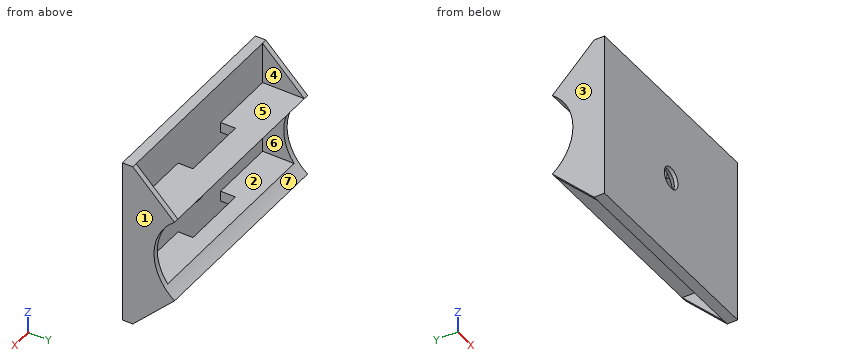
```python
from build123d import *

# Parameters (mm, degrees)
SKETCH4_W           = 25.4
SKETCH4_H           = 1.5875
SKETCH4_W_2         = 1.5875
SKETCH4_H_2         = 6.35
BOSS_EXTRUDE2_DEPTH = 31.75
SKETCH5_W           = 9.525
SKETCH5_H           = 6.35
BOSS_EXTRUDE3_DEPTH = 0.79375
BOSS_EXTRUDE4_DEPTH = 0.79375
SKETCH7_W           = 10.16
SKETCH7_H           = 2.260476196
CUT_EXTRUDE1_DEPTH  = 38.867781903
CUT_EXTRUDE2_REACH  = 43.427
SKETCH8_R           = 8.011204241


with BuildPart() as part:
    # Sketch4 → Boss-Extrude2 (new body)
    with BuildSketch(Plane(origin=(0, 0, 0), x_dir=(0, 0, -1), z_dir=(1, 0, 0))):
        with Locations((12.7, 0.79375)):
            Rectangle(SKETCH4_W, SKETCH4_H)
        with Locations((7.14375, 4.7625)):
            Rectangle(SKETCH4_W_2, SKETCH4_H_2)
        with Locations((18.25625, 4.7625)):
            Rectangle(SKETCH4_W_2, SKETCH4_H_2)
    extrude(amount=BOSS_EXTRUDE2_DEPTH)

    # Sketch5 → Boss-Extrude3 (add)
    with BuildSketch(Plane(origin=(31.75, 0, 0), x_dir=(0, 0, -1), z_dir=(1, 0, 0))):
        Polygon((6.35, 7.9375), (0, 1.5875), (6.35, 1.5875), align=None)
        with Locations((12.7, 4.7625)):
            Rectangle(SKETCH5_W, SKETCH5_H)
        Polygon((19.05, 7.9375), (19.05, 1.5875), (25.4, 1.5875), align=None)
    extrude(amount=-BOSS_EXTRUDE3_DEPTH)

    # Sketch6 → Boss-Extrude4 (add)
    with BuildSketch(Plane.ZY):
        Polygon((-25.4, 1.5875), (0, 1.5875), (-6.35, 7.9375), (-19.05, 7.9375), align=None)
    extrude(amount=-BOSS_EXTRUDE4_DEPTH)

    # Sketch7 → Cut-Extrude1 (cut, through all)
    with BuildSketch(Plane.XY.offset(-6.35)):
        with Locations((15.875, 2.717738098)):
            Rectangle(SKETCH7_W, SKETCH7_H)
    extrude(amount=-CUT_EXTRUDE1_DEPTH, mode=Mode.SUBTRACT)

    # Sketch8 → Cut-Extrude2 (cut, up to next)
    with BuildSketch(Plane(origin=(31.75, 0, 0), x_dir=(0, 0, -1), z_dir=(1, 0, 0)), mode=Mode.PRIVATE) as cut_extrude2_sk1:
        with Locations((12.7, 12.82185189)):
            Circle(SKETCH8_R)
    cut_extrude2_tool1 = extrude(cut_extrude2_sk1.sketch, amount=-CUT_EXTRUDE2_REACH, mode=Mode.PRIVATE) & part.part
    add(cut_extrude2_tool1.solids().sort_by_distance((31.75, 12.821852, -12.7))[0], mode=Mode.SUBTRACT)

    # Sketch10 → CSK for #4 Flat Head Machine Screw (100)1 (revolve, cut)
    with BuildSketch(Plane(origin=(15.887282669, 1.5875, -12.697770178), x_dir=(0, 0, 1), z_dir=(1, 0, 0))):
        Polygon((0, 0), (0, 1.5875), (1.63195, 1.5875), (1.63195, 1.028358553), (2.8575, 0), align=None)
    revolve(axis=Axis((15.887282669, 7.9375, -12.697770178), (0, -1, 0)), mode=Mode.SUBTRACT)


solid = part.part
```
The listing builds one solid part. Answer for the finished solid, in the listing's coordinates (mm). Face numbers are marked on the shaded views. A direction names the side the tool comes from. Round coordinates to 2 decimals unless told otherwise and drop trailing zeros. Loops run counter-clockwise (first coordinate to the right, second up) from the corner with the lowest first, then second, coordinate; pieces in that order, holes last. Notation, with made-up numbers: (18.25, 28.5) - (30.25, 28.5) arc R29 ccw to (30.25, 57.5) - close; hole circle Ø11 at (-39, -18.5). An arc over 180 degrees is marked (long way). Return JSON: item names as keys, results as strings. Group by question number.
1. The part is cut by section A-A on y = 6. Determine the outline of the cut face in (x, z).
2. The part is cut by section B-B on x = 20. Determine the outline of the cut face in (y, z), then the cut area to 3 significant figures.
3. The mould has two halves that part along X. Classify the marked faces 1, 2, 3 and 4: pulls with the +X half, pulls with the -X half, needs draft (parallel to the pull), parting line crosses it, or undercut.
4. Each of these flat-tipped pins is pushed along its axis until it touches: P1, Ø3, axis at x = 4.5, z = -12.5, coming from the -Y side; P2, Ø2, axis at x = 22.5, y = 4.5, coming from the -Z side; P3, Ø3, axis at x = 13.5, y = 5.5, coming from the +Z side. Where does it stop, or does it pass through?
5. Which of the six approach directions +Z, -Z, +X, -X, +Y, -Y give full straight-line access (tool end or side, diameter ignored) to the marked faces 5, 6 and 7?
6. The part is cut by section C-C on x = 6.5. Determine the outline of the cut face in (y, z), then the cut area to 3 significant figures.
7. Consider probe 1 along Z at (x, y) = (6, 4); probe 2 along X at (y, z) = (2.25, -18) (3 decimals); probe 3 along X at (y, z) = (5.5, -16.25). Determine where each line is inside the solid, lowest interval first.
Resolved:
{
 "1": {"outline": "(0, -20.99) - (0.79, -20.99) - (0.79, -19.05) - (30.96, -19.05) - (30.96, -20.99) - (31.75, -20.99) - (31.75, -16.9) - (30.96, -16.9) - (30.96, -17.46) - (0.79, -17.46) - (0.79, -16.9) - (0, -16.9) - close; (0, -8.5) - (0.79, -8.5) - (0.79, -7.94) - (30.96, -7.94) - (30.96, -8.5) - (31.75, -8.5) - (31.75, -4.41) - (30.96, -4.41) - (30.96, -6.35) - (0.79, -6.35) - (0.79, -4.41) - (0, -4.41) - close"},
 "2": {"outline": "(0, -25.4) - (1.59, -25.4) - (1.59, 0) - (0, 0) - close; (3.85, -19.05) - (7.94, -19.05) arc R8.01 cw to (6.38, -17.46) - (3.85, -17.46) - close; (3.85, -7.94) - (6.38, -7.94) arc R8.01 cw to (7.94, -6.35) - (3.85, -6.35) - close", "area": "50.6 mm²"},
 "3": {"face 1": "pulls with the +X half", "face 2": "undercut", "face 3": "pulls with the -X half", "face 4": "undercut"},
 "4": {"P1": "stops at y = 0", "P2": "stops at z = -19.05", "P3": "stops at z = -6.35"},
 "5": {"face 5": "+Z, +Y", "face 6": "+Y", "face 7": "+X, -X, +Y"},
 "6": {"outline": "(0, -25.4) - (1.59, -25.4) - (1.59, -19.05) - (7.94, -19.05) arc R8.01 cw to (6.38, -17.46) - (1.59, -17.46) - (1.59, -7.94) - (6.38, -7.94) arc R8.01 cw to (7.94, -6.35) - (1.59, -6.35) - (1.59, 0) - (0, 0) - close", "area": "57.8 mm²"},
 "7": {"probe 1": "z = -19.05 to -17.46, -7.94 to -6.35", "probe 2": "x = 0 to 10.795, 20.955 to 31.75", "probe 3": "x = 0 to 0.79, 30.96 to 31.75"}
}
